The listing builds one solid part. Answer for the finished solid, in the listing's coordinates (mm). Face numbers are marked on the shaded views. A direction names the side the tool comes from. Give positions to 0.01 mm unless a question says otherwise; leave off trailing zeros. Order: outer loops, then holes, each group sorted by start corner. A loop starts at its lowest first (then second) coordinate and runs counter-clockwise, first axis right, second up. Notation, with made-up numbers: (74.5, 49) - (87.5, 49) arc R17 ccw to (87.5, 81) - close; hole circle Ø6 at (54.25, 57). An arc over 180 degrees is marked (long way). Answer in a Markdown table with one row per item. Add a question column.
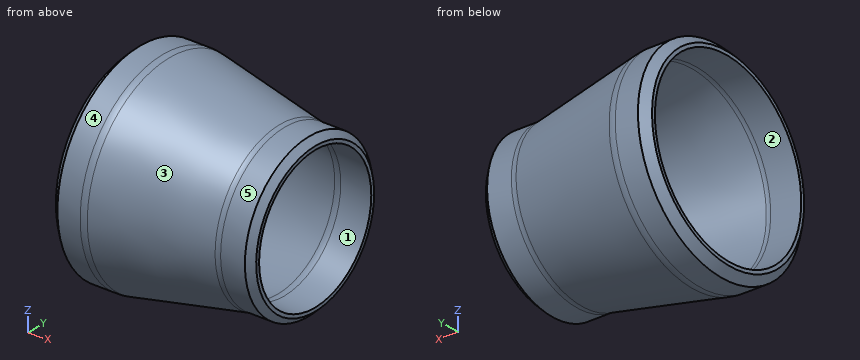
```python
from build123d import *

# Parameters (mm, degrees)
F4_SIZE = 3.5
F5_SIZE = 4.35


with BuildPart() as f3:
    # F2 (on Front) → F3 (revolve)
    with BuildSketch(Plane.XZ):
        with BuildLine():
            Line((0, 57.15), (0, 50.8))
            Line((0, 50.8), (17, 50.8))
            ThreePointArc((17, 50.8), (18.1432578461, 50.7484371168), (19.2772322795, 50.5941671649))
            Line((19.2772322795, 50.5941671649), (81.3570260515, 39.2792785118))
            ThreePointArc((81.3570260515, 39.2792785118), (83.1710875139, 39.0324870796), (85, 38.95))
            Line((85, 38.95), (102, 38.95))
            Line((102, 38.95), (102, 44.45))
            Line((102, 44.45), (85, 44.45))
            ThreePointArc((85, 44.45), (83.5664884716, 44.5195091165), (82.1464269481, 44.7273842927))
            Line((82.1464269481, 44.7273842927), (20.6688796382, 56.7933630522))
            ThreePointArc((20.6688796382, 56.7933630522), (18.8430862508, 57.0606311359), (17, 57.15))
            Line((17, 57.15), (0, 57.15))
        make_face()
    revolve(axis=Axis((51, 0, 0), (-1, 0, 0)))

    # F4
    f4_edges = [f3.edges().sort_by_distance(p)[0] for p in [
        (102, 0, -44.45),
    ]]
    chamfer(f4_edges, length=F4_SIZE)

    # F5
    f5_edges = [f3.edges().sort_by_distance(p)[0] for p in [
        (0, 0, -57.15),
    ]]
    chamfer(f5_edges, length=F5_SIZE)


solid = f3.part
```
(1) Straight lines are drawn through the part: line 1 (Y direction, x = 92.5, z = 0); line 2 (Y direction, x = 4, z = 0); line 3 (Z direction, x = 92, y = 22). For each, find the intervals that lie inside material, in ascending order.
(2) For the marked faces 4 and 5, determine the directions among +Z, -Z, +X, -X, +Y, -Y from which every point of the face is accessible in a straight line to the end or side of a thin tool.
(3) Find section A-A, the plane y = 0. Write down the section's boundary in (x, z), plus the area to 3 significant figures.
(4) Find section C-C, the plane x = 31. Write down the section's boundary in (y, z), plus the area to 3 significant figures.
(5) The mould has two halves that part along Z. Classify the marked faces 1, 2 and 3: +Z half, -Z half, draft (parallel to the pull), parting line (faces both ways), or undercut.
(6) Find section D-D, the plane x = 14. Write down the section's boundary in (y, z).
(7) Each of these flat-tipped pins is pushed along its axis until it touches: P1, Ø3, axis at x = 40, y = -33, coming from the +Z side; P2, Ø6, axis at x = 77.5, z = 18.5, coming from the -Y side; P3, Ø1, axis at x = 18, z = 31.5, coming from the +Y side. Where does it stop, or does it pass through?
Answer key:
| question | item | result |
|---|---|---|
| 1 | line 1 | -44.45 to -38.95, 38.95 to 44.45 |
| 1 | line 2 | -56.8 to -50.8, 50.8 to 56.8 |
| 1 | line 3 | -38.62 to -32.14, 32.14 to 38.62 |
| 2 | face 4 | +X, -X |
| 2 | face 5 | +X |
| 3 | outline | (0, -52.8) - (4.35, -57.15) - (17, -57.15) arc R19.05 ccw to (20.67, -56.79) - (82.15, -44.73) arc R14.82 cw to (85, -44.45) - (98.5, -44.45) - (102, -40.95) - (102, -38.95) - (85, -38.95) arc R20.32 ccw to (81.36, -39.28) - (19.28, -50.59) arc R12.7 cw to (17, -50.8) - (0, -50.8) - close; (0, 50.8) - (17, 50.8) arc R12.7 cw to (19.28, 50.59) - (81.36, 39.28) arc R20.32 ccw to (85, 38.95) - (102, 38.95) - (102, 40.95) - (98.5, 44.45) - (85, 44.45) arc R14.82 cw to (82.15, 44.73) - (20.67, 56.79) arc R19.05 ccw to (17, 57.15) - (4.35, 57.15) - (0, 52.8) - close |
| 3 | area | 1,190 mm² |
| 4 | outline | circle Ø109.53 at (0, 0); hole circle Ø96.92 at (0, 0) |
| 4 | area | 2,050 mm² |
| 5 | face 1 | undercut |
| 5 | face 2 | undercut |
| 5 | face 3 | parting line |
| 6 | outline | circle Ø114.3 at (0, 0); hole circle Ø101.6 at (0, 0) |
| 7 | P1 | z = 42.68 |
| 7 | P2 | y = -43.09 |
| 7 | P3 | y = 47.98 |
